Work out the finished part from the listing and answer in its coordinate system (mm). Face numbers are marked on the shaded views. A direction names the side the tool comes from. Give positions to 0.01 mm unless a question says otherwise; leave off trailing zeros. Write each loop counter-clockwise with the first axis right and the second up, starting at its lowest first coordinate (ties: lowest second). Pieces come first, ordered by that corner, then holes. Notation, with made-up numbers: (-25, 54) -> (14, 54) arc R12 cw to (14, 68) -> close; hole circle Ø5 at (-14.5, 22). An arc over 180 degrees is marked (long way). Use a Markdown table: item, result. Add a question column.
Q1. Consider line 1 (Y direction, x = 16, z = -25); line 2 (Y direction, x = 19.55, z = -25); line 3 (X direction, y = 1, z = -15). Determine where each line is inside the solid, lowest interval first.
Q2. Section A-A, the plane x = 17 is taken. Give the vertices of the cut face in (y, z), plus the area to 3 significant figures.
Q3. Section C-C, the plane z = -25 is taken. Give the vertices of the cut face in (x, y) (3 decimals).
Q4. Each of these flat-tipped pins is pushed along its axis until it touches: pin 1 Ø8 at (x, z) = (7, -35) entering from -Y; pin 2 Ø7 at (y, z) = (-17, -25) entering from -X; pin 3 Ø9 at (y, z) = (-17, -26.5) entering from -X; pin 4 Ø3.5 at (y, z) = (-27, -25) entering from -X. Where does it stop, or does it pass through?
Q5. Section D-D, the plane y = 1 is taken. Give the vertices of the cut face in (x, z).
Q6. Section B-B, the plane y = -17 is taken. Give the vertices of the cut face in (x, z) (3 decimals), plus the area to 3 significant figures.
Q7. For the marked faces 1 and 2, determine the directions among +Z, -Z, +X, -X, +Y, -Y from which every point of the face is accessible in a straight line to the end or side of a thin tool.
from build123d import *

# Parameters (mm, degrees)
ESBO_O1_W                                    = 15
ESBO_O1_H                                    = 50
RESSALTO_EXTRUS_O1_DEPTH                     = 5
ESBO_O2_R                                    = 2.5
CORTE_EXTRUS_O1_DEPTH                        = 53.440442409
FILETE1_R                                    = 10
RESSALTO_EXTRUS_O2_DEPTH                     = 6
REBAIXO_PARA_PARAFUSO_COM_CABE_A_RED_2_COUNT = 2
REBAIXO_PARA_PARAFUSO_COM_CABE_A_RED_2_PITCH = 10


with BuildPart() as part:
    # Esboço1 → Ressalto-extrusão1 (new body)
    with BuildSketch(Plane(origin=(0, 0, 0), x_dir=(1, 0, 0), z_dir=(0, 1, 0))):
        with Locations((7.5, 25)):
            Rectangle(ESBO_O1_W, ESBO_O1_H)
    extrude(amount=RESSALTO_EXTRUS_O1_DEPTH)

    # Esboço2 → Corte-extrusão1 (cut, through all)
    with BuildSketch(Plane(origin=(0, 5, 0), x_dir=(1, 0, 0), z_dir=(0, 1, 0))):
        with Locations(Location((7, 35, 0), (0, 0, 270))):
            Circle(ESBO_O2_R)
        with Locations(Location((7, 15, 0), (0, 0, 270))):
            Circle(ESBO_O2_R)
    extrude(amount=-CORTE_EXTRUS_O1_DEPTH, mode=Mode.SUBTRACT)

    # Filete1
    filete1_edges = [part.edges().sort_by_distance(p)[0] for p in [
        (0, 2.5, -50),
        (0, 2.5, 0),
    ]]
    fillet(filete1_edges, radius=FILETE1_R)

    # Esboço3 → Ressalto-extrusão2 (add)
    with BuildSketch(Plane(origin=(15, 0, 0), x_dir=(0, 0, -1), z_dir=(1, 0, 0))):
        Polygon((50, 5), (0, 5), (0, 0), (17, -32.5), (33, -32.5), (50, 0), align=None)
    extrude(amount=RESSALTO_EXTRUS_O2_DEPTH)

    # Esboço6 → Rebaixo para parafuso com cabeça redonda de M41 (revolve, cut)
    with BuildSketch(Plane(origin=(15, -27, -25), x_dir=(0, 0, 1), z_dir=(0, 1, 0))):
        Polygon((0, 0), (0, 6), (2.25, 6), (2.25, 2.6), (4, 2.6), (4, 0.025), (4.025, 0), align=None)
    rebaixo_para_parafuso_com_cabe_a_redonda = revolve(axis=Axis((8.65, -27, -25), (1, 0, 0)), mode=Mode.SUBTRACT)

    # Rebaixo para parafuso com cabe_a red 2: Rebaixo para parafuso com cabeça redonda de M41 ×2
    with Locations(*[(0, i * REBAIXO_PARA_PARAFUSO_COM_CABE_A_RED_2_PITCH, 0) for i in range(1, REBAIXO_PARA_PARAFUSO_COM_CABE_A_RED_2_COUNT)]):
        add(rebaixo_para_parafuso_com_cabe_a_redonda, mode=Mode.SUBTRACT)


solid = part.part
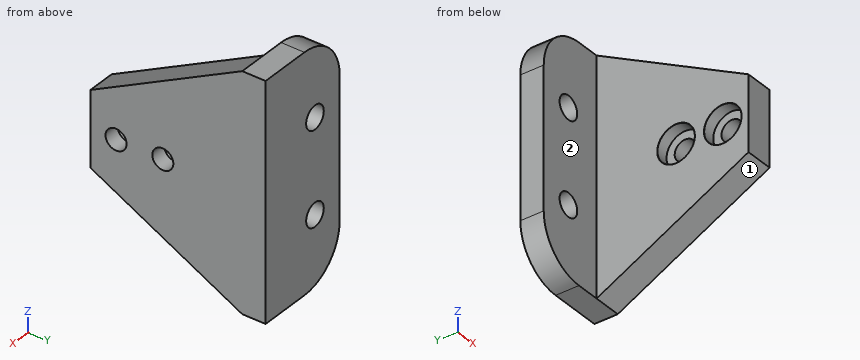
Result set:
| question | item | result |
|---|---|---|
| 1 | line 1 | y = -32.5 to -31, -23 to -21, -13 to 5 |
| 1 | line 2 | y = -32.5 to -29.25, -24.75 to -19.25, -14.75 to 5 |
| 1 | line 3 | x = 0 to 4.5, 9.5 to 21 |
| 2 | outline | (-32.5, -33) -> (0, -50) -> (5, -50) -> (5, 0) -> (0, 0) -> (-32.5, -17) -> close; hole circle Ø8 at (-27, -25); hole circle Ø8 at (-17, -25) |
| 2 | area | 1,220 mm2 |
| 3 | outline | (0, 0) -> (15, 0) -> (15, -12.975) -> (15.025, -13) -> (17.6, -13) -> (17.6, -14.75) -> (21, -14.75) -> (21, 5) -> (0, 5) -> close; (15, -32.5) -> (21, -32.5) -> (21, -29.25) -> (17.6, -29.25) -> (17.6, -31) -> (15.025, -31) -> (15, -31.025) -> close; (15, -22.975) -> (15.025, -23) -> (17.6, -23) -> (17.6, -24.75) -> (21, -24.75) -> (21, -19.25) -> (17.6, -19.25) -> (17.6, -21) -> (15.025, -21) -> (15, -21.025) -> close |
| 4 | pin 1 | stops at y = 0 |
| 4 | pin 2 | stops at x = 17.6 |
| 4 | pin 3 | stops at x = 15 |
| 4 | pin 4 | passes through |
| 5 | outline | (0, -40) arc R10 ccw to (10, -50) -> (21, -50) -> (21, 0) -> (10, 0) arc R10 ccw to (0, -10) -> close; hole circle Ø5 at (7, -35); hole circle Ø5 at (7, -15) |
| 6 | outline | (15, -41.108) -> (21, -41.108) -> (21, -27.25) -> (17.6, -27.25) -> (17.6, -29) -> (15.025, -29) -> (15, -29.025) -> close; (15, -20.975) -> (15.025, -21) -> (17.6, -21) -> (17.6, -22.75) -> (21, -22.75) -> (21, -8.892) -> (15, -8.892) -> close |
| 6 | area | 157 mm2 |
| 7 | face 1 | -Z, +X, -X, -Y |
| 7 | face 2 | +Z, -Z, -X, -Y |
